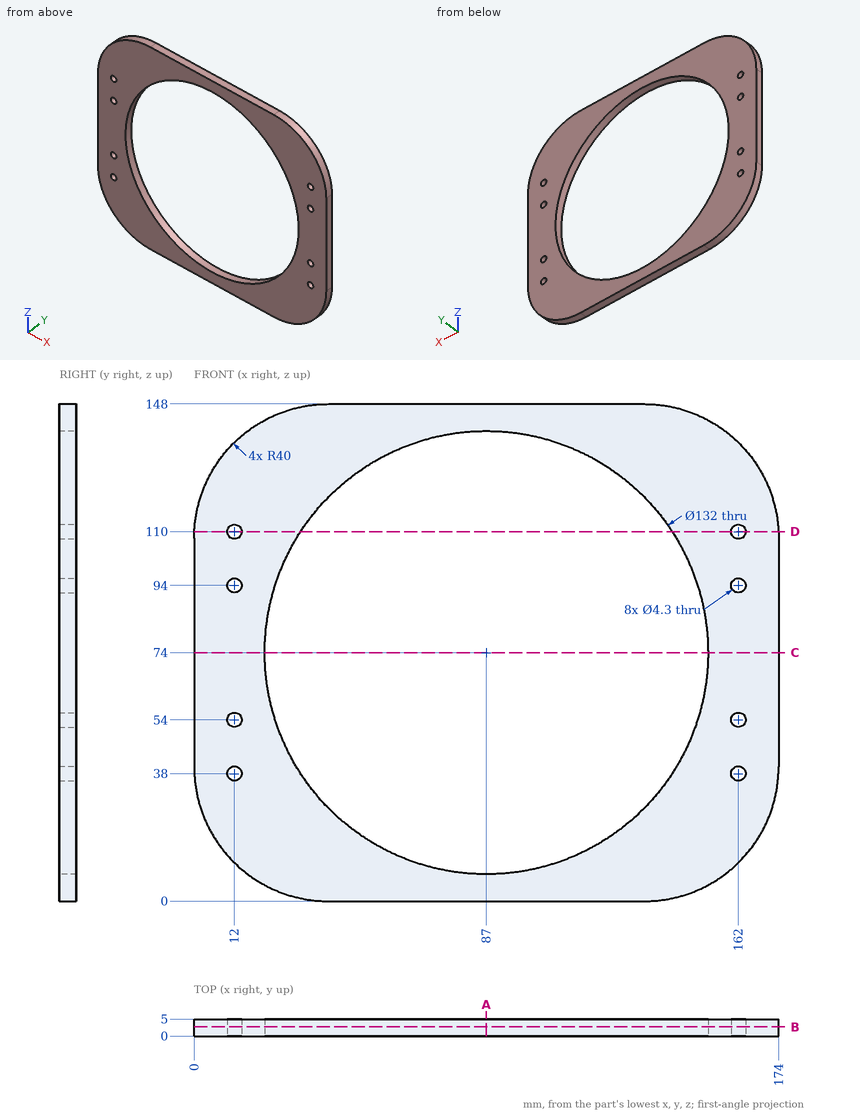
For this review, use the dimensioned drawing (mm, ordinates from the lowest corner) and the shaded views. Round coordinates to 2 decimals unless told otherwise and drop trailing zeros. Order: outer loops, then holes, each group sorted by start corner. A loop starts at its lowest first (then second) coordinate and runs counter-clockwise, first axis right, second up. Notation, with made-up numbers: M 21,83 L 70,83 A31 cw 70,121 Z; hole C 58.5,-20 d9. An arc over 180 degrees is marked long. Write each question's results on one line, items separated by ' | '. Start each with the question number.
1. To check wall thickness, follow L1, parallel to X at y = 1.7, z = 74; L2, parallel to X at y = 2.8, z = 94; L3, parallel to X at y = 3.2, z = 110. State the ranges of each line that lie inside material, in increasing order. Write a range as [from, to].
2. Add section D-D (z = 110). State the section outline as (x, y) points, then the cut area to 3 significant figures.
3. Add section B-B (y = 2.7). State how many separate pieces and enclosed holes the cut face has, then the cut area to 3 significant figures.
4. Clearance check with a flat-ended pin moving along its axis: pin 1 Ø4 at (x, z) = (12, 54) entering from +Y. State where the tip first meets the part, or that it passes through.
5. Add section A-A (x = 87). State the section outline as (y, z) points, then the cut area to 3 significant figures.
6. Add section C-C (z = 74). State the section outline as (x, y) points, then the cut area to 3 significant figures.
Output values:
1) L1: [0, 21], [153, 174] | L2: [0, 9.85], [14.15, 24.1], [149.9, 159.85], [164.15, 174] | L3: [0.05, 9.85], [14.15, 31.68], [142.32, 159.85], [164.15, 173.95]
2) outline: M 0.05,0 L 9.85,0 L 9.85,5 L 0.05,5 Z; M 14.15,0 L 31.68,0 L 31.68,5 L 14.15,5 Z; M 142.32,0 L 159.85,0 L 159.85,5 L 142.32,5 Z; M 164.15,0 L 173.95,0 L 173.95,5 L 164.15,5 Z | area: 273 mm^2
3) separate pieces: 1 | enclosed holes: 9 | area: 10,600 mm^2
4) pin 1: through
5) outline: M 0,0 L 5,0 L 5,8 L 0,8 Z; M 0,140 L 5,140 L 5,148 L 0,148 Z | area: 80.0 mm^2
6) outline: M 0,0 L 21,0 L 21,5 L 0,5 Z; M 153,0 L 174,0 L 174,5 L 153,5 Z | area: 210 mm^2
